Geometry check sheet. Reference: the model listing, model coordinates, mm. A direction names the side the tool comes from. Coordinates: 2 decimals unless noted, no trailing zeros. Write each loop counter-clockwise with the first axis right and the second up, starting at its lowest first coordinate (ties: lowest second). Pieces come first, ordered by that corner, then holes. Notation, with made-up numbers: M 18,9 L 75,9 A25 ccw 75,30 Z; hole C 29.25,-32 d11. An arc over 180 degrees is marked long. Write item = value, one per line. Start each with the question number.
```python
from build123d import *

# Parameters (mm, degrees)
BOSS_EXTRUDE1_DEPTH      = 150
BOSS_EXTRUDE1_DEPTH_BACK = 150
CUT_EXTRUDE1_DEPTH       = 399.19822728
CUT_EXTRUDE1_DEPTH_BACK  = 399.19822728
SKETCH2_OUTSIDE_W        = 417.444
SKETCH2_OUTSIDE_H        = 376.444
CUT_EXTRUDE2_DEPTH       = 399.198227346
CUT_EXTRUDE2_DEPTH_BACK  = 399.198227346
SKETCH3_W                = 4
SKETCH3_H                = 11
SKETCH3_H_2              = 18.5
CUT_EXTRUDE3_DEPTH       = 399.198227346
CUT_EXTRUDE3_DEPTH_BACK  = 399.198227346
SKETCH4_R                = 2
CUT_EXTRUDE4_DEPTH       = 399.198227346
CUT_EXTRUDE4_DEPTH_BACK  = 399.198227346
SKETCH6_W                = 17
SKETCH6_H                = 54


with BuildPart() as part:
    # Sketch1 → Boss-Extrude1 (new, two sides: drawn at the far end of the back side and taken through both)
    with BuildSketch(Plane(origin=(0, 0, 0), x_dir=(0, 0, -1), z_dir=(1, 0, 0)).offset(-BOSS_EXTRUDE1_DEPTH_BACK)):
        with BuildLine():
            Line((-152, 0), (-152, 254))
            Line((-152, 254), (152, 254))
            Line((152, 254), (152, 0))
            Line((152, 0), (157, 0))
            Line((157, 0), (157, 259))
            Line((157, 259), (-157, 259))
            Line((-157, 259), (-157, 31.183582697))
            ThreePointArc((-157, 31.183582697), (-165.22850184, 12.643980503), (-184.497347959, 6.308630372))
            ThreePointArc((-184.497347959, 6.308630372), (-222.45464291, 12.402261203), (-259.428077267, 22.930970935))
            Line((-259.428077267, 22.930970935), (-262.642015315, 19.100748719))
            ThreePointArc((-262.642015315, 19.100748719), (-208.13932257, 4.810245455), (-152, 0))
        make_face()
    extrude(amount=BOSS_EXTRUDE1_DEPTH + BOSS_EXTRUDE1_DEPTH_BACK)

    # Sketch2 outside → Cut-Extrude1 (cut, two sides: drawn at the far end of the back side and taken through both)
    with BuildSketch(Plane.XY.offset(-CUT_EXTRUDE1_DEPTH_BACK)):
        with Locations((0, 129.5)):
            Rectangle(SKETCH2_OUTSIDE_W, SKETCH2_OUTSIDE_H)
        with BuildLine():
            ThreePointArc((0, 0), (56.126949793, 13.395552699), (103.124452968, 46.875547032))
            ThreePointArc((103.124452968, 46.875547032), (136.604447301, 93.873050207), (150, 150))
            ThreePointArc((150, 150), (137.347558964, 204.051684319), (106.180566109, 249.989548857))
            ThreePointArc((106.180566109, 249.989548857), (57.545132629, 283.138396945), (0, 295.5))
            ThreePointArc((0, 295.5), (-57.545132629, 283.138396945), (-106.180566109, 249.989548857))
            ThreePointArc((-106.180566109, 249.989548857), (-137.347558964, 204.051684319), (-150, 150))
            ThreePointArc((-150, 150), (-136.604447301, 93.873050207), (-103.124452968, 46.875547032))
            ThreePointArc((-103.124452968, 46.875547032), (-56.126949793, 13.395552699), (0, 0))
        make_face(mode=Mode.SUBTRACT)
    extrude(amount=CUT_EXTRUDE1_DEPTH + CUT_EXTRUDE1_DEPTH_BACK, mode=Mode.SUBTRACT)

    # Sketch3 → Cut-Extrude2 (cut, two sides: drawn at the far end of the back side and taken through both)
    with BuildSketch(Plane(origin=(0, 0, 0), x_dir=(0, 0, -1), z_dir=(1, 0, 0)).offset(-CUT_EXTRUDE2_DEPTH_BACK)):
        with Locations((-152, 198)):
            Rectangle(SKETCH3_W, SKETCH3_H)
        with Locations((152, 198)):
            Rectangle(SKETCH3_W, SKETCH3_H_2)
    extrude(amount=CUT_EXTRUDE2_DEPTH + CUT_EXTRUDE2_DEPTH_BACK, mode=Mode.SUBTRACT)

    # Sketch4 → Cut-Extrude3 (cut, two sides: drawn at the far end of the back side and taken through both)
    with BuildSketch(Plane.XY.offset(-CUT_EXTRUDE3_DEPTH_BACK)):
        with Locations((-120, 198)):
            Circle(SKETCH4_R)
        with Locations((120, 198)):
            Circle(SKETCH4_R)
        with Locations((40, 198)):
            Circle(SKETCH4_R)
        with Locations((-40, 198)):
            Circle(SKETCH4_R)
    extrude(amount=CUT_EXTRUDE3_DEPTH + CUT_EXTRUDE3_DEPTH_BACK, mode=Mode.SUBTRACT)

    # Sketch6 → Cut-Extrude4 (cut, two sides: drawn at the far end of the back side and taken through both)
    with BuildSketch(Plane.XY.offset(-CUT_EXTRUDE4_DEPTH_BACK)):
        with Locations((-127.5, 143.5)):
            Rectangle(SKETCH6_W, SKETCH6_H)
        with Locations((127.5, 143.5)):
            Rectangle(SKETCH6_W, SKETCH6_H)
    extrude(amount=CUT_EXTRUDE4_DEPTH + CUT_EXTRUDE4_DEPTH_BACK, mode=Mode.SUBTRACT)


solid = part.part
```
Q1. Cross-section at C-C on y = 181. Enter the section's corners in (x, z).
Q2. Scan lines: L1, parallel to Z at x = 80, y = 69; L2, parallel to Y at x = 120, z = 156.15; L3, parallel to X at y = 198, z = -155.7. Record each from-to range of solid material in increasing order.
Q3. Draft check along Z on faces 1 (the face through (55.386, 13.061, -154.535)), 2 (the face through (-2, 128, -157)), 3 (the face through (-2, 116, 152)). Enter one of: pulls with the +Z half, pulls with the -Z half, needs draft (parallel to the pull), parting line crosses it, or undercut.
Q4. Gauge pin test, flat ends, axial feed: pin 1 (1 mm diameter, centred on x = -95.5, z = 21, fed in from -Y); pin 2 (3.5 mm diameter, centred on x = 40, y = 198, fed in from -Z) (3 decimals); pin 3 (23.5 mm diameter, centred on x = -62, y = 222.5, fed in from +Z); pin 4 (2.5 mm diameter, centred on x = -124.5, z = -155, fed in from -Y). Record the tip position at first contact, or that the pin passes through.
Q5. Set-up check for faces 4 (the face through (-1.2, 16.29, 161.92)), 5 (the face through (-2, 198, -154)), 6 (the face through (-2, 147, 157)), 7 (the face through (-1, 254, 2)): record each of +Z, -Z, +X, -X, +Y, -Y from which the full face is reachable in a straight line by a thin tool's end or side.
Q6. Cross-section at A-A on y = 124. Enter the section's corners in (x, z), and give its area (3 significant figures).
Q7. Cross-section at B-B on x = -51.5. Enter the section's corners in (y, z).
Q8. Cross-section at D-D on z = 53. Enter the section's corners in (x, y).
Values found:
q1.outline = M -145.32,-157 L 145.32,-157 L 145.32,-152 L -145.32,-152 Z; M -145.32,152 L 145.32,152 L 145.32,157 L -145.32,157 Z
q2.L1 = -157 to -152, 152 to 157
q2.L2 = 65.84 to 116.5, 170.5 to 196, 200 to 233.9
q2.L3 = -139.85 to -122, -118 to -42, -38 to 38, 42 to 118, 122 to 139.85
q3.face_1 = needs draft
q3.face_2 = pulls with the -Z half
q3.face_3 = undercut
q4.pin_1 = 254
q4.pin_2 = through
q4.pin_3 = 157
q4.pin_4 = 70.35
q5.face_4 = +X, -X, +Y
q5.face_5 = +X, -X
q5.face_6 = +Z, +X, -X, +Y
q5.face_7 = +X, -X, -Y
q6.outline = M -146.63,-157 L -136,-157 L -136,-152 L -146.63,-152 Z; M -146.63,152 L -136,152 L -136,157 L -146.63,157 Z; M -119,-157 L 119,-157 L 119,-152 L -119,-152 Z; M -119,152 L 119,152 L 119,157 L -119,157 Z; M 136,-157 L 146.63,-157 L 146.63,-152 L 136,-152 Z; M 136,152 L 146.63,152 L 146.63,157 L 136,157 Z
q6.area = 2,590 mm²
q7.outline = M 11.38,-157 L 259,-157 L 259,157 L 31.18,157 A25 cw 11.38,166.74 L 11.38,152 L 192.5,152 L 192.5,154 L 203.5,154 L 203.5,152 L 254,152 L 254,-152 L 207.25,-152 L 207.25,-154 L 188.75,-154 L 188.75,-152 L 11.38,-152 Z; M 11.38,217.7 A325.32 cw 22.93,259.43 L 19.1,262.64 A330 ccw 11.38,237.93 Z
q8.outline = M -102.07,254 L 102.07,254 A153.18 ccw 96.48,259 L -96.48,259 A153.18 ccw Z
